For this review, take the finished solid that the model builds, in its own axes (mm). Face numbers are marked on the shaded views. A direction names the side the tool comes from. Give positions to 0.01 mm unless a question says otherwise; leave off trailing zeros. Loops run counter-clockwise (first coordinate to the right, second up) from the corner with the lowest first, then second, coordinate; pieces in that order, holes last. Notation, with made-up numbers: (-10, 69) - (16, 69) arc R10 ccw to (16, 86) - close; hole circle Ø4 at (54.25, 3.5). An arc over 180 degrees is marked (long way). Use CSV: the item, a comma, the result in double quotes. Start each with the question number.
1. Take a section at D-D on y = 10. Give the boundary of the cut face in (x, z), plus the area to 3 significant figures.
2. For pin 1 (1 mm diameter, centred on x = 5, z = 1.5, fed in from +Y); pin 2 (1.5 mm diameter, centred on y = 1, z = -0.5, fed in from -X); pin 3 (1.5 mm diameter, centred on y = -9, z = 3.5, fed in from +X), all flat-tipped, find the tip position at first contact; note any pin that passes through.
3. Take a section at C-C on z = -1.75. Give the boundary of the cut face in (x, y).
4. Take a section at A-A on x = 2.5. Give the boundary of the cut face in (y, z).
5. Take a section at B-B on y = -3.5. Give the boundary of the cut face in (x, z), plus the area to 3 significant figures.
6. Wall thickness on line 1 (Y direction, x = -6.5, z = -2.5); line 2 (X direction, y = -5.5, z = -2.25); line 3 (X direction, y = 7, z = -1.75): over which ranges is each line inside the solid? List them lowest first.
7. Mouldability with a two-part tool opening along X and no side actions: class the marked faces 1, 2 and 3 as pulls with the +X half, pulls with the -X half, needs draft (parallel to the pull), parting line crosses it, or undercut.
8. For the marked faces 4 and 5, list the 3-axis set-ups (+Z, -Z, +X, -X, +Y, -Y) from which the entire face can be reached by the end or side of a thin tool; tool diameter is ignored.
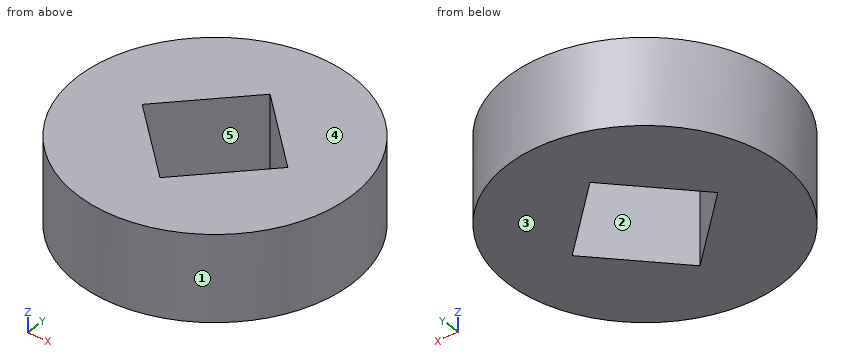
Autodesk Inventor part; units mm, degrees
ref_plane "YZ Plane" through (0, 0, 0) normal (1, 0, 0) x (0, 1, 0)
ref_plane "XZ Plane" through (0, 0, 0) normal (0, 1, 0) x (-1, 0, 0)
ref_plane "XY Plane" through (0, 0, 0) normal (0, 0, 1) x (1, 0, 0)
sketch "Эскиз1" plane through (0, 0, 0) normal (0, 0, 1) x (1, 0, 0)
  circle A0 centre (0, 0) radius 16
  line L0 (0, 8.4853) -> (8.4853, 0)
  line L1 (8.4853, 0) -> (0, -8.4853)
  line L2 (0, -8.4853) -> (-8.4853, 0)
  line L3 (-8.4853, 0) -> (0, 8.4853)
  dimension "d0" = 32
  dimension "d1" = 12
extrude "Выдавливание1" add sketch "Эскиз1" along normal mid plane 10
properties part number "7"
Check result:
1,outline,"(-12.49, -5) - (12.49, -5) - (12.49, 5) - (-12.49, 5) - close"
1,area,"250 mm²"
2,pin 1,"stops at y = 15.35"
2,pin 2,"stops at x = -16"
2,pin 3,"stops at x = 13.71"
3,outline,"circle Ø32 at (0, 0); hole (-8.49, 0) - (0, -8.49) - (8.49, 0) - (0, 8.49) - close"
4,outline,"(-15.8, -5) - (-5.99, -5) - (-5.99, 5) - (-15.8, 5) - close; (5.99, -5) - (15.8, -5) - (15.8, 5) - (5.99, 5) - close"
5,outline,"(-15.61, -5) - (-4.99, -5) - (-4.99, 5) - (-15.61, 5) - close; (4.99, -5) - (15.61, -5) - (15.61, 5) - (4.99, 5) - close"
5,area,"213 mm²"
6,line 1,"y = -14.62 to -1.99, 1.99 to 14.62"
6,line 2,"x = -15.02 to -2.99, 2.99 to 15.02"
6,line 3,"x = -14.39 to -1.49, 1.49 to 14.39"
7,face 1,"parting line crosses it"
7,face 2,"undercut"
7,face 3,"needs draft"
8,face 4,"+Z, +X, -X, +Y, -Y"
8,face 5,"+Z, -Z"
